Could you check a few things on this model? Use its own coordinates, in mm. Round coordinates to 2 decimals unless told otherwise and drop trailing zeros. Loops run counter-clockwise (first coordinate to the right, second up) from the corner with the lowest first, then second, coordinate; pieces in that order, holes last. Notation, with made-up numbers: M 20,-17.5 L 40,-17.5 A17 ccw 40,-12.5 Z; hole C 56,-31.75 d3. An arc over 180 degrees is marked long. One line per item, written item: value. Start each with the question number.
Q1. Imagine slicing it at B-B (y = 141). Please give me the cut outline in (x, z), then the cut area to 3 significant figures.
Q2. Please list where these lines run through material, in increasing order: line 1 along X through (y, z) = (-37, 3) (3 decimals); line 2 along Y through (x, z) = (38.1, 2.75); line 3 along X through (y, z) = (29.5, 5.25).
Q3. Imagine slicing it at A-A (z = 1.5). Please give me the cut outline in (x, y) (3 decimals), then the cut area to 3 significant figures.
Q4. Imagine slicing it at C-C (x = 329). Please give me the cut outline in (y, z).
Q5. I'm going to push flat-ended pins straight in: pin 1 Ø1.9 at (y, z) = (128, 2) entering from +X; pin 2 Ø3 at (x, z) = (221.5, 4.5) entering from +Y; pin 3 Ø5.5 at (x, y) = (38.1, 12.75) entering from +Z; pin 4 Ø8.5 at (x, y) = (38.1, 127.05) entering from +Z. Where does each tip first touch, or does it pass through?
from build123d import *

# Parameters (mm, degrees)
F0_W     = 76.2
F0_H     = 76.2
F1_DEPTH = 6.35
F2_R     = 3.175
F3_DEPTH = 25.4


# Not quite as in the source:
# - a feature names something its author has since deleted; it is built from what else it names


with BuildPart() as f1:
    # F0 (on Top) → F1 (new body)
    with BuildSketch(Plane.XY):
        with BuildLine():
            Line((0, 0), (76.2, 0))
            Line((76.2, 0), (76.2, 171.45))
            ThreePointArc((76.2, 171.45), (74.3401280605, 175.9401280605), (69.85, 177.8))
            Line((69.85, 177.8), (6.35, 177.8))
            ThreePointArc((6.35, 177.8), (1.8598719395, 175.9401280605), (0, 171.45))
            Line((0, 171.45), (0, 0))
        make_face()
        with Locations((38.1, -38.1)):
            Rectangle(F0_W, F0_H)
        Polygon((111.125, -38.1), (111.125, 0), (76.2, 0), (76.2, -76.2), (250.825, -76.2), (257.175, -76.2), (381, -76.2), (381, 0), (346.075, 0), (346.075, -38.1), (342.9, -38.1), (339.725, -38.1), (339.725, 0), (257.175, 0), (250.825, 0), (117.475, 0), (117.475, -38.1), (114.3, -38.1), align=None)
    extrude(amount=F1_DEPTH)

    # F2 (on face) → F3 (cut)
    with BuildSketch(Plane.XY.offset(6.35)):
        with Locations((38.1, 12.7454660833)):
            Circle(F2_R)
        with Locations((38.1, 50.8454660833)):
            Circle(F2_R)
        with Locations((38.1, 88.9454660833)):
            Circle(F2_R)
        with Locations((38.1, 127.0454660833)):
            Circle(F2_R)
        with Locations((38.1, 165.1454660833)):
            Circle(F2_R)
    extrude(amount=-F3_DEPTH, mode=Mode.SUBTRACT)


solid = f1.part
Report:
1. outline: M 0,0 L 76.2,0 L 76.2,6.35 L 0,6.35 Z
1. area: 484 mm²
2. line 1: x = 0 to 111.125, 117.475 to 339.725, 346.075 to 381
2. line 2: y = -76.2 to 9.57, 15.92 to 47.67, 54.02 to 85.77, 92.12 to 123.87, 130.22 to 161.97, 168.32 to 177.8
2. line 3: x = 0 to 76.2
3. outline: M 0,-76.2 L 381,-76.2 L 381,0 L 346.075,0 L 346.075,-38.1 L 339.725,-38.1 L 339.725,0 L 117.475,0 L 117.475,-38.1 L 111.125,-38.1 L 111.125,0 L 76.2,0 L 76.2,171.45 A6.35 ccw 69.85,177.8 L 6.35,177.8 A6.35 ccw 0,171.45 Z; hole C 38.1,12.745 d6.35; hole C 38.1,50.845 d6.35; hole C 38.1,88.945 d6.35; hole C 38.1,127.045 d6.35; hole C 38.1,165.145 d6.35
3. area: 41,900 mm²
4. outline: M -76.2,0 L 0,0 L 0,6.35 L -76.2,6.35 Z
5. pin 1: stops at x = 76.2
5. pin 2: stops at y = 0
5. pin 3: passes through
5. pin 4: stops at z = 6.35
